Autodesk Inventor part; units mm, degrees
ref_plane "Work Plane1" through (15, 0, 0) normal (1, 0, 0) x (0, 0, -1)
ref_plane "YZ Plane" through (0, 0, 0) normal (1, 0, 0) x (0, 1, 0)
ref_plane "XZ Plane" through (0, 0, 0) normal (0, 1, 0) x (-1, 0, 0)
sketch "Sketch1" plane through (0, 0, 0) normal (0, 0, 1) x (1, 0, 0)
  line L0 (0, 0) -> (30, 0)
  line L1 (30, 0) -> (30, 50)
  line L2 (30, 50) -> (0, 50)
  line L3 (0, 50) -> (0, 0)
  dimension "d0" = 30
  dimension "d1" = 50
extrude "Extrusion1" add sketch "Sketch1" along normal blind 3
ref_plane "Work Plane1" through (15, 0, 0) normal (1, 0, 0) x (0, 0, -1)
sketch "Sketch4" plane through (0, 0, 0) normal (0, 0, -1) x (-1, 0, 0)
  line L0 (-28, 30) -> (-28, 20) construction
  line L1 (-29, 29) -> (-29, 21)
  line L2 (-27, 21) -> (-27, 29)
  arc A0 (-27, 29) -> (-29, 29) centre (-28, 29) ccw
  arc A1 (-29, 21) -> (-27, 21) centre (-28, 21) ccw
  line L3 (-2, 30) -> (-2, 20) construction
  line L4 (-3, 29) -> (-3, 21)
  line L5 (-1, 21) -> (-1, 29)
  arc A2 (-1, 29) -> (-3, 29) centre (-2, 29) ccw
  arc A3 (-3, 21) -> (-1, 21) centre (-2, 21) ccw
  line L6 (-30, 0) -> (-30, 50)
  point P0 (0, 0)
  point P1 (-28, 25)
  point P2 (-2, 25)
  dimension "d19" = 25
  dimension "d20" = 1
  dimension "d21" = 1
  dimension "d22" = 10
  dimension "d23" = 10
  dimension "d25" = 1
  dimension "d29" = 1
extrude "Extrusion4" add sketch "Sketch4" along normal blind 3.5
properties part number "motor box"
Geometry: final body of the model. Coordinates: model frame, mm. A direction names the side the tool comes from. Give positions to 0.01 mm unless a question says otherwise; leave off trailing zeros. Order: outer loops, then holes, each group sorted by start corner. A loop starts at its lowest first (then second) coordinate and runs counter-clockwise, first axis right, second up. Notation, with made-up numbers: (11, 37.5) -> (41, 37.5) arc R20 cw to (41, 53.5) -> close; hole circle Ø8 at (-21, 37). An arc over 180 degrees is marked (long way). Write each question's results on one line, items separated by ' | '. Start each with the question number.
1) Draft query along X for faces 1 (the flat face through (15, 0, 1)), 2 (the flat face through (30, 25, 1)), 3 (the flat face through (0, 25, 1)), 4 (the cylindrical face through (28, 30, -2)). Return one class per face: pulls with the +X half, pulls with the -X half, needs draft (parallel to the pull), parting line crosses it, or undercut.
2) First-contact query: pin 1 (1 mm diameter, centred on y = 27, z = -2, fed in from -X); pin 2 (1.8 mm diameter, centred on y = 26.5, z = -2.5, fed in from +X); pin 3 (1.5 mm diameter, centred on x = 23.5, z = -1, fed in from +Y); pin 4 (10 mm diameter, centred on x = 23.5, y = 44.5, fed in from -Z). Flat tips, straight axial feed; report the tip coordinate or a pass-through.
3) Section C-C (x = 28). Return loops of the section in (y, z), then the cut area to 3 significant figures.
4) Set-up query: faces 5 (the flat face through (29, 25, -2)), 6 (the cylindrical face through (2, 30, -2)), 7 (the flat face through (27, 25, -2)), 8 (the cylindrical face through (28, 20, -2)). Return all of +Z, -Z, +X, -X, +Y, -Y with unobstructed straight access to the full face (end or side cutting, diameter ignored); none if empty.
5) Line query: line 1 (X direction, y = 27, z = -0.25); line 2 (Z direction, x = 19.5, y = 41.5); line 3 (Y direction, x = 2, z = -0.25). Output: solid intervals per line, ascending. Write a range as from..to.
6) Section B-B (y = 27.5). Return loops of the section in (x, z), then the cut area to 3 significant figures.
7) Section D-D (x = 17.25). Return loops of the section in (y, z), then the cut area to 3 significant figures.
8) Section A-A (z = -0.5). Return loops of the section in (x, y), then the cut area to 3 significant figures.
Calculated:
1) face 1: needs draft | face 2: pulls with the +X half | face 3: pulls with the -X half | face 4: undercut
2) pin 1: x = 1 | pin 2: x = 29 | pin 3: through | pin 4: z = 0
3) outline: (0, 0) -> (20, 0) -> (20, -3.5) -> (30, -3.5) -> (30, 0) -> (50, 0) -> (50, 3) -> (0, 3) -> close | area: 185 mm2
4) face 5: -Z, +X, +Y, -Y | face 6: -Z, +Y | face 7: -Z, +Y, -Y | face 8: -Z, -Y
5) line 1: 1..3, 27..29 | line 2: 0..3 | line 3: 20..30
6) outline: (0, 0) -> (1, 0) -> (1, -3.5) -> (3, -3.5) -> (3, 0) -> (27, 0) -> (27, -3.5) -> (29, -3.5) -> (29, 0) -> (30, 0) -> (30, 3) -> (0, 3) -> close | area: 104 mm2
7) outline: (0, 0) -> (50, 0) -> (50, 3) -> (0, 3) -> close | area: 150 mm2
8) outline: (1, 21) arc R1 ccw to (3, 21) -> (3, 29) arc R1 ccw to (1, 29) -> close; (27, 21) arc R1 ccw to (29, 21) -> (29, 29) arc R1 ccw to (27, 29) -> close | area: 38.3 mm2
